Verification items for the finished model (mm, model axes). Face numbers are marked on the shaded views. A direction names the side the tool comes from. Round coordinates to 2 decimals unless told otherwise and drop trailing zeros. Order: outer loops, then holes, each group sorted by start corner. A loop starts at its lowest first (then second) coordinate and runs counter-clockwise, first axis right, second up. Notation, with made-up numbers: M -28,60 L -15,60 A26 ccw -15,94 Z; hole C 16,35.5 d7. An arc over 180 degrees is marked long. Use one line per item in the form item = value. Start each with the question number.
Item 1: Go/stop test with flat-tipped pins: pin 1 Ø2.5 at (x, y) = (-16, 7.5) entering from +Z; pin 2 Ø3 at (x, y) = (-16.5, 5) entering from +Z (3 decimals). Record where each tip stops, or that it passes through.
Item 2: Cross-section at C-C on y = 4.75. Enter the section's corners in (x, z) (3 decimals).
Item 3: Thickness scan on probe 1 along Z at (x, y) = (-23, 8.25); probe 2 along Z at (x, y) = (-7.75, 6.25); probe 3 along Y at (x, z) = (-6.5, -4). Record the ranges inside material, lowest first. Write a range as [from, to].
Item 4: Cross-section at D-D on x = -4.5. Enter the section's corners in (y, z) (3 decimals), then the cut area to 3 significant figures.
Item 5: Tool access check on the marked faces 1 and 2. Record the directions out of +Z, -Z, +X, -X, +Y, -Y that give a thin tool (end or side, any length) a straight path to the whole face; none if there is none.
Item 6: Cross-section at A-A on z = -17. Enter the section's corners in (x, y), then the cut area to 3 significant figures.
Item 7: Cross-section at B-B on x = -13. Enter the section's corners in (y, z) (3 decimals).
Autodesk Inventor part; units mm, degrees
ref_plane "YZ Plane" through (0, 0, 0) normal (1, 0, 0) x (0, 1, 0)
ref_plane "XZ Plane" through (0, 0, 0) normal (0, 1, 0) x (-1, 0, 0)
ref_plane "XY Plane" through (0, 0, 0) normal (0, 0, 1) x (1, 0, 0)
sketch "Sketch1" plane through (0, 0, 0) normal (0, 1, 0) x (-1, 0, 0)
  line L0 (0, 0) -> (25.4, 0)
  line L1 (25.4, 0) -> (25.4, -25.4)
  line L2 (25.4, -25.4) -> (0, -25.4)
  line L3 (0, -25.4) -> (0, 0)
  dimension "d0" = 25.4
  dimension "d1" = 25.4
extrude "Extrusion1" add sketch "Sketch1" along normal blind 2.54
sketch "Sketch2" plane through (0, 2.54, 0) normal (0, 1, 0) x (1, 0, 0)
  line L0 (0, 25.4) -> (-25.4, 25.4)
  line L1 (-25.4, 25.4) -> (0, 25.4)
  line L2 (0, 25.4) -> (0, 24.13)
  line L3 (0, 24.13) -> (-25.4, 24.13)
  line L4 (-25.4, 24.13) -> (-25.4, 25.4)
  line L5 (-12.7, 24.13) -> (-12.7, 16.51)
  line L6 (-12.7, 24.13) -> (-5.08, 24.13) construction
  line L7 (-25.4, 16.51) -> (0, 16.51)
  line L8 (0, 16.51) -> (0, 13.97)
  line L9 (0, 13.97) -> (-25.4, 13.97)
  line L10 (-25.4, 13.97) -> (-25.4, 16.51)
  point P0 (0, 0)
  dimension "d4" = 25.4
  dimension "d5" = 1.27
  dimension "d6" = 7.62
  dimension "d7" = 90
  dimension "d8" = 25.4
  dimension "d9" = 2.54
extrude "Extrusion2" add sketch "Sketch2" along normal blind 3.81
sketch "Sketch3" plane through (0, 6.35, 0) normal (0, 1, 0) x (1, 0, 0)
  line L0 (0, 13.97) -> (0, 16.51)
  line L1 (-25.4, 25.4) -> (0, 25.4)
  line L2 (0, 13.97) -> (-25.4, 13.97)
  line L3 (-25.4, 13.97) -> (-25.4, 25.4)
  line L4 (-25.4, 25.4) -> (0, 25.4)
  line L5 (0, 25.4) -> (0, 13.97)
  point P0 (0, 0)
extrude "Extrusion3" add sketch "Sketch3" along normal blind 2.54
chamfer "Chamfer1" distance 3.175 angle 45 1 edges at (-12.7, 2.54, -13.97)
sketch "Sketch4" plane through (0, 8.89, 0) normal (0, 1, 0) x (1, 0, 0)
  circle A0 centre (-20.546, 20.0791) radius 1.27
  circle A1 centre (-4.3777, 20.0791) radius 1.27
  point P0 (0, 0)
  dimension "d17" = 2.54
  dimension "d18" = 2.54
extrude "Extrusion4" cut sketch "Sketch4" against normal blind 25.4
sketch "Sketch5" plane through (-25.4, 0, 0) normal (0, 0, 1) x (1, 0, 0)
  line L0 (0, 2.54) -> (25.4, 2.54)
  line L1 (25.4, 0) -> (0, 0)
  line L2 (0, 2.54) -> (25.4, 2.54)
  line L3 (25.4, 2.54) -> (25.4, 0)
  line L4 (25.4, 0) -> (0, 0)
  line L5 (0, 0) -> (0, 2.54)
extrude "Extrusion5" add sketch "Sketch5" along normal blind 12.7
sketch "Sketch6" plane through (0, 0, -25.4) normal (0, 0, -1) x (-1, 0, 0)
  line L0 (25.4, 0) -> (0, 0)
  line L1 (25.4, 0) -> (25.4, 8.89)
  line L2 (0, 8.89) -> (25.4, 8.89)
  line L3 (0, 0) -> (0, 8.89)
extrude "Extrusion6" add sketch "Sketch6" along normal blind 1.27
properties part number "Hotend holder V4 Beltmount"
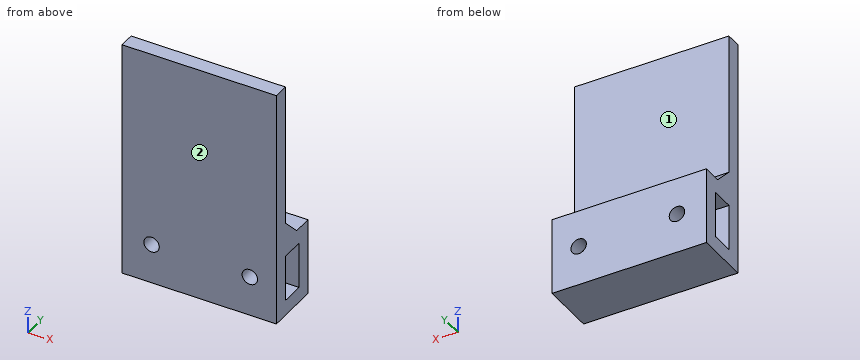
Output values:
q1.pin_1 = -13.97
q1.pin_2 = -11.755
q2.outline = M -25.4,-26.67 L 0,-26.67 L 0,-24.13 L -25.4,-24.13 Z; M -25.4,-16.51 L 0,-16.51 L 0,-13.005 L -25.4,-13.005 Z
q3.probe_1 = [-26.67, -13.97]
q3.probe_2 = [-26.67, -24.13], [-16.51, -13.97]
q3.probe_3 = [0, 2.54]
q4.outline = M 0,-26.67 L 8.89,-26.67 L 8.89,-21.343 L 6.35,-21.343 L 6.35,-24.13 L 2.54,-24.13 L 2.54,-21.343 L 0,-21.343 Z; M 0,-18.815 L 2.54,-18.815 L 2.54,-16.51 L 6.35,-16.51 L 6.35,-18.815 L 8.89,-18.815 L 8.89,-13.97 L 5.715,-13.97 L 2.54,-10.795 L 2.54,12.7 L 0,12.7 Z
q4.area = 144 mm2
q5.face_1 = +Z, +X, -X, +Y
q5.face_2 = +Z, -Z, +X, -X, -Y
q6.outline = M -25.4,0 L 0,0 L 0,2.54 L -25.4,2.54 Z; M -25.4,6.35 L 0,6.35 L 0,8.89 L -25.4,8.89 Z
q6.area = 129 mm2
q7.outline = M 0,-26.67 L 8.89,-26.67 L 8.89,-13.97 L 5.715,-13.97 L 2.54,-10.795 L 2.54,12.7 L 0,12.7 Z; hole M 2.54,-24.13 L 6.35,-24.13 L 6.35,-16.51 L 2.54,-16.51 Z
